Verification items for the finished model (mm, model axes). A direction names the side the tool comes from. Round coordinates to 2 decimals unless told otherwise and drop trailing zeros. Use a Markdown table: item, result. Add a question column.
from build123d import *

# Parameters (mm, degrees)
F1_ANGLE_BACK = 50
F1_ANGLE      = 100
F2_SIZE       = 5
F3_R          = 1.5
F4_DEPTH      = 3.7476667667


with BuildPart() as f1:
    # F0 (on Front) → F1 (revolve)
    with BuildSketch(Plane.XZ, mode=Mode.PRIVATE) as f1_sk:
        Polygon((3, 0), (7, 75), (-3, 75), (-3, 65), (2.1333333333, 65), (0, 25), (0, 0), align=None)
    revolve(f1_sk.sketch.rotate(Axis((1.5, 0, 0), (-1, 0, 0)), -F1_ANGLE_BACK), axis=Axis((1.5, 0, 0), (-1, 0, 0)), revolution_arc=F1_ANGLE)

    # F2
    f2_edges = [f1.edges().sort_by_distance(p)[0] for p in [
        (-3, 0, 75),
    ]]
    chamfer(f2_edges, length=F2_SIZE)

    # F3 (on Right) → F4 (cut, through all)
    with BuildSketch(Plane.YZ):
        with Locations((0, 12.5)):
            Circle(F3_R)
    extrude(amount=F4_DEPTH, mode=Mode.SUBTRACT)


solid = f1.part
1. Depth check by flat-ended pin: pin 1 Ø1 at (x, z) = (6, 59) entering from -Y; pin 2 Ø1 at (y, z) = (-18, 51.5) entering from +X; pin 3 Ø6 at (x, y) = (0, 13.5) entering from +Z; pin 4 Ø2.5 at (y, z) = (0, 12.5) entering from +X. Enter the tip coordinate at first touch or a pass-through.
2. Access from +Z, -Z, +X, -X, +Y, -Y to the whole of each face (thin tool, end or side, straight path). Record for faces 5 (the conical face through (4.584, -0.363, 29.689)), 6 (the conical face through (-2.757, -0.858, 70.238)), 7 (the cylindrical face through (-0.397, -0.794, 64.995)).
3. Release check for a two-part mould opening along Y. For faces 1 (the conical face through (0.815, -0.492, 40.273)), 2 (the flat face through (3.041, 35.513, 29.799)), 3 (the flat face through (3.041, -35.513, 29.799)), 4 (the flat face through (0, 0, 16)) record: +Y half, -Y half, draft (parallel to the pull), parting line (faces both ways), or undercut.
4. Scan lines: line 1 along Z through (x, y) = (2.9, 0); line 2 along Y through (x, z) = (2.1, 12.5); line 3 along Y through (x, z) = (1.25, 49). Record each from-to range of solid material in increasing order. Write a range as from..to.
Answer:
| question | item | result |
|---|---|---|
| 1 | pin 1 | stops at y = -46.93 |
| 1 | pin 2 | stops at x = 5.94 |
| 1 | pin 3 | stops at z = 74.15 |
| 1 | pin 4 | passes through |
| 2 | face 5 | -Z, +X |
| 2 | face 6 | +Z, -X |
| 2 | face 7 | -X |
| 3 | face 1 | undercut |
| 3 | face 2 | +Y half |
| 3 | face 3 | -Y half |
| 3 | face 4 | draft |
| 4 | line 1 | z = 0..11, 14..75 |
| 4 | line 2 | y = -14.9..-1.5, 1.5..14.9 |
| 4 | line 3 | y = -55.79..-42.71, 42.71..55.79 |
